Answer from the drawing. Dimensions are ordinates in mm from the lowest x, y and z of the part. A direction names the side the tool comes from. Coordinates: 2 decimals unless noted, no trailing zeros. Write each loop counter-clockwise with the first axis right and the second up, starting at its lowest first coordinate (ties: lowest second). Pieces come first, ordered by that corner, then holes. Notation, with made-up numbers: (48.25, 29) -> (61.25, 29) arc R19 cw to (61.25, 59) -> close; hole circle Ø4 at (-22, -13.75). An arc over 180 degrees is marked (long way). Return JSON: item names as keys, results as strings.
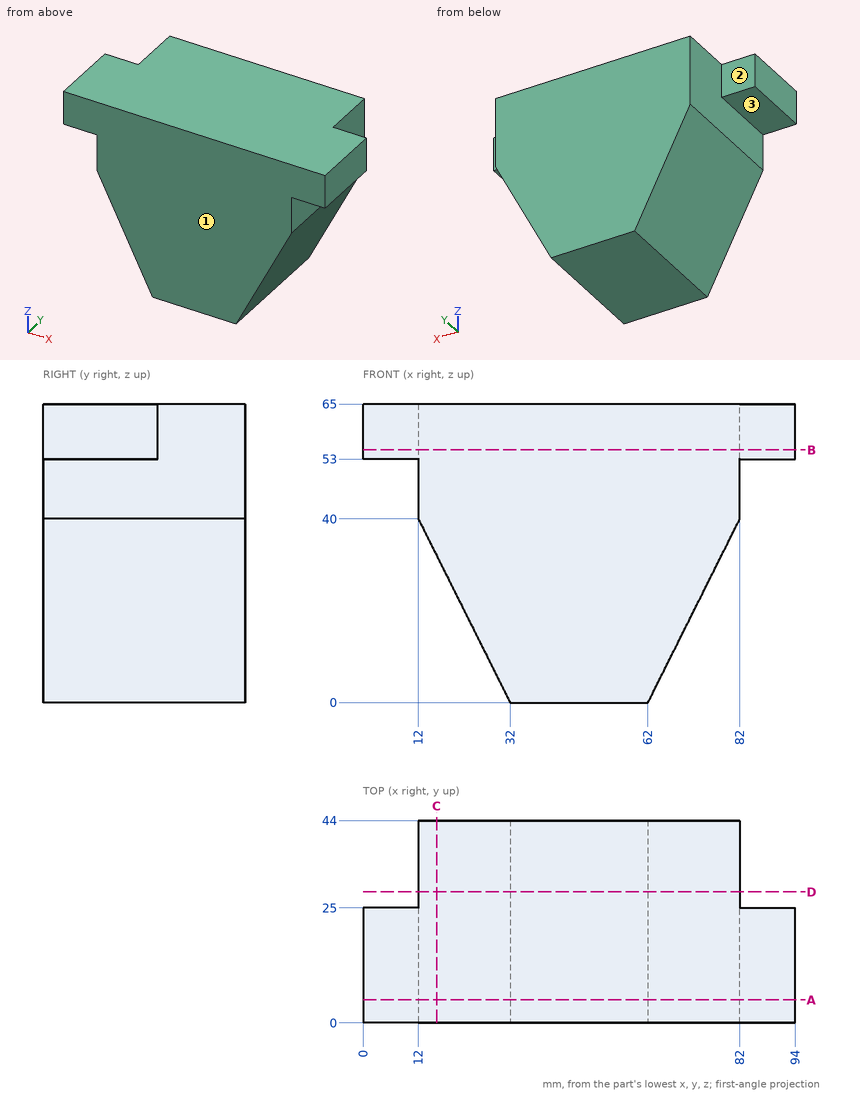
1. A tool of negligible diameter and unlimited length cuts with its end or side. For the marked faces 1, 2 and 3, from which of +Z, -Z, +X, -X, +Y, -Y can it reach the whole face along a straight path? Write none if from no direction.
Taken from the geometry:
{"face 1": "+Z, -Z, +X, -X, -Y", "face 2": "+Z, -Z, -X, +Y", "face 3": "-Z, -X, +Y, -Y"}
2. The part is cut by section C-C (x = 16). Determine the outline of the cut face in (y, z), then the cut area to 3 significant figures.
Taken from the geometry:
{"outline": "(0, 32) -> (44, 32) -> (44, 65) -> (0, 65) -> close", "area": "1,450 mm2"}
3. The part is cut by section B-B (z = 55). Determine the outline of the cut face in (x, y), then the cut area to 3 significant figures.
Taken from the geometry:
{"outline": "(0, 0) -> (94, 0) -> (94, 25) -> (82, 25) -> (82, 44) -> (12, 44) -> (12, 25) -> (0, 25) -> close", "area": "3,680 mm2"}
4. The part is cut by section A-A (y = 5). Determine the outline of the cut face in (x, z), then the cut area to 3 significant figures.
Taken from the geometry:
{"outline": "(0, 53) -> (12, 53) -> (12, 40) -> (32, 0) -> (62, 0) -> (82, 40) -> (82, 53) -> (94, 53) -> (94, 65) -> (0, 65) -> close", "area": "4,040 mm2"}
5. Flat-ended cylindrical pins translate along their axes: pin 1 Ø2 at (x, y) = (73, 16.5) entering from -Z; pin 2 Ø12.5 at (y, z) = (27, 49) entering from +X; pin 3 Ø3.5 at (x, z) = (91, 61) entering from +Y; pin 4 Ø10 at (y, z) = (4.5, 12.5) entering from +X. Find the tip coordinate at first contact, or state that the pin passes through.
Taken from the geometry:
{"pin 1": "stops at z = 20", "pin 2": "stops at x = 94", "pin 3": "stops at y = 25", "pin 4": "stops at x = 70.75"}
6. The part is cut by section D-D (y = 28.5). Determine the outline of the cut face in (x, z), then the cut area to 3 significant figures.
Taken from the geometry:
{"outline": "(12, 40) -> (32, 0) -> (62, 0) -> (82, 40) -> (82, 65) -> (12, 65) -> close", "area": "3,750 mm2"}
7. Consider L1, parallel to X at y = 27.5, z = 44; L2, parallel to Z at x = 6, y = 24; L3, parallel to X at y = 29, z = 36.5. Determine where each line is inside the solid, lowest interval first.
Taken from the geometry:
{"L1": "x = 12 to 82", "L2": "z = 53 to 65", "L3": "x = 13.75 to 80.25"}
